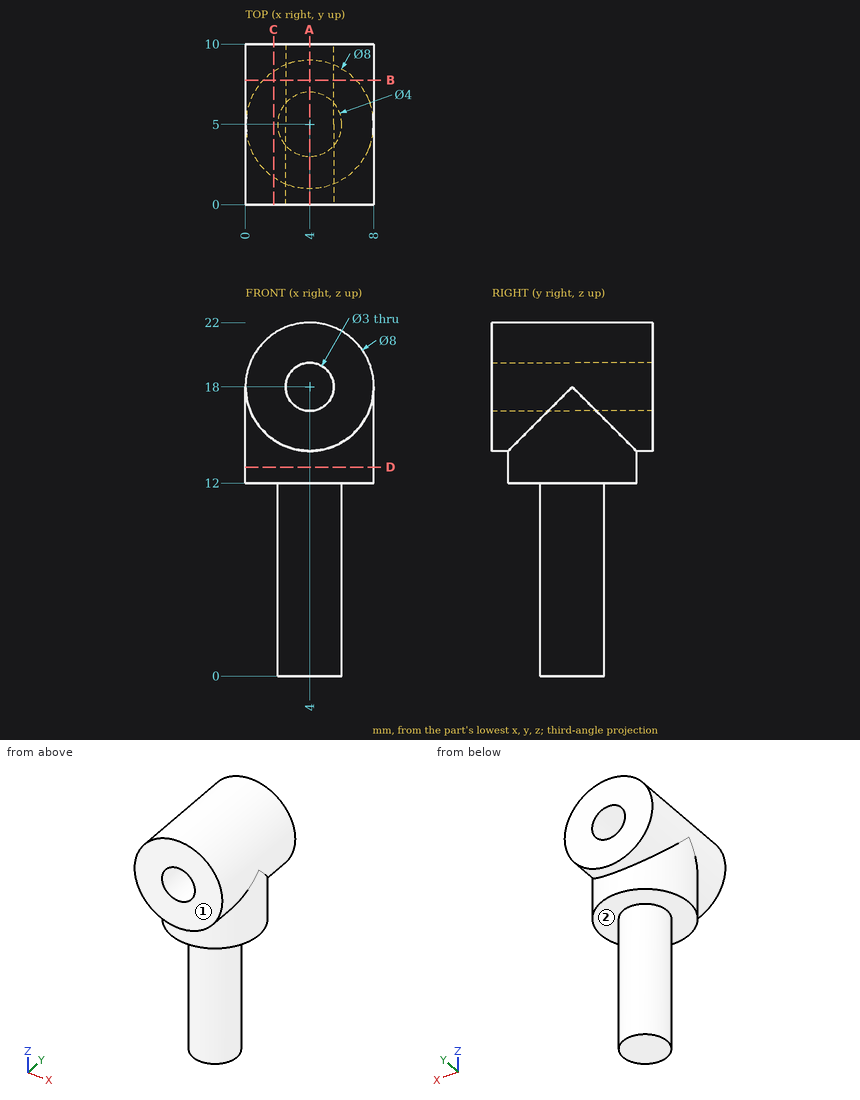
Answer from the drawing. Dimensions are ordinates in mm from the lowest x, y and z of the part. A direction names the side the tool comes from. Round coordinates to 2 decimals unless told otherwise and drop trailing zeros. Loops run counter-clockwise (first coordinate to the right, second up) from the corner with the lowest first, then second, coordinate; pieces in that order, holes last. Notation, with made-up numbers: (48, 39.5) - (71, 39.5) arc R26 ccw to (71, 55.5) - close; hole circle Ø11 at (-38.75, -31.5). An arc over 180 degrees is marked (long way). One line per item, written item: value.
Q1. For the marked faces 1 and 2, determine the directions among +Z, -Z, +X, -X, +Y, -Y from which every point of the face is accessible in a straight line to the end or side of a thin tool.
Check values:
face 1: +Z, -Z, +X, -X, -Y
face 2: -Z
Q2. Each of these flat-tipped pins is pushed along its axis until it touches: pin 1 Ø1 at (x, y) = (5.5, 8.5) entering from -Z; pin 2 Ø3 at (x, y) = (2, 6.5) entering from +Z; pin 3 Ø2 at (x, y) = (1, 6) entering from +Z. Where does it stop, or does it pass through?
Check values:
pin 1: z = 12
pin 2: z = 21.97
pin 3: z = 21.46
Q3. Find section D-D on z = 13. Give the vertices of the cut face in (x, y), and give its area (3 significant figures).
Check values:
outline: circle Ø8 at (4, 5)
area: 50.3 mm2
Q4. Find section A-A on x = 4. Give the vertices of the cut face in (y, z), and give its area (3 significant figures).
Check values:
outline: (0, 14) - (1, 14) - (1, 12) - (3, 12) - (3, 0) - (7, 0) - (7, 12) - (9, 12) - (9, 14) - (10, 14) - (10, 16.5) - (0, 16.5) - close; (0, 19.5) - (10, 19.5) - (10, 22) - (0, 22) - close
area: 114 mm2
Q5. Straight lines are drawn through the part: probe 1 along X at (y, z) = (2.2, 18); probe 2 along Z at (x, y) = (4, 7.3); probe 3 along Z at (x, y) = (4, 4). For each, find the intervals that lie inside material, in ascending order.
Check values:
probe 1: 0 to 2.5, 5.5 to 8
probe 2: 12 to 16.5, 19.5 to 22
probe 3: 0 to 16.5, 19.5 to 22
Q6. Find section B-B on y = 7.75. Give the vertices of the cut face in (x, z), and give its area (3 significant figures).
Check values:
outline: (1.1, 12) - (6.9, 12) - (6.9, 15.25) arc R4 ccw (long way) to (1.1, 15.25) - close; hole circle Ø3 at (4, 18)
area: 57.1 mm2
Q7. Find section C-C on x = 1.75. Give the vertices of the cut face in (y, z).
Check values:
outline: (0, 14.69) - (1.69, 14.69) - (1.69, 12) - (8.31, 12) - (8.31, 14.69) - (10, 14.69) - (10, 21.31) - (0, 21.31) - close
